Check sheet for the drawn part. Datum: minimum x, y, z corner. Units: mm. A direction names the side the tool comes from. Round coordinates to 2 decimals unless told otherwise and drop trailing zeros. Write each loop counter-clockwise with the first axis right and the second up, starting at its lowest first coordinate (ties: lowest second). Pieces come first, ordered by that corner, then holes. Notation, with made-up numbers: (3.5, 86.5) - (9.5, 86.5) arc R19 cw to (9.5, 117.5) - close; hole circle Ø5 at (15, 6.5). An arc over 180 degrees is marked (long way). Answer as a JSON object with one key per item and string values.
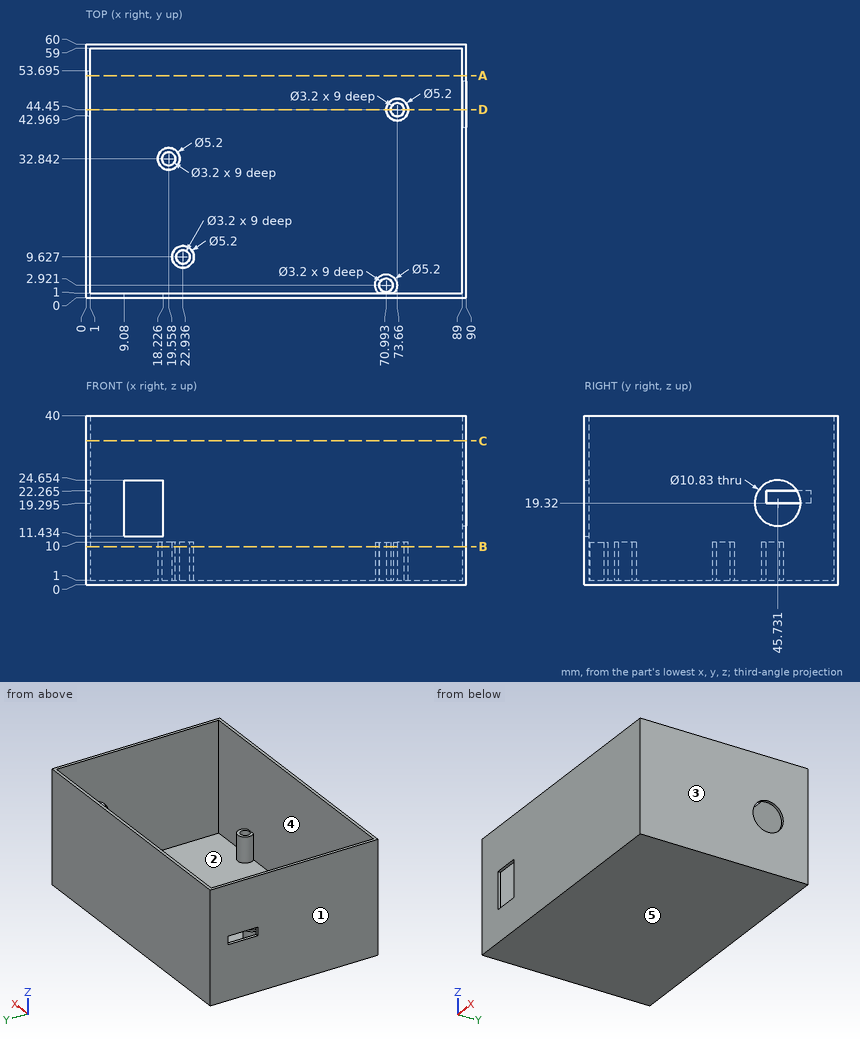
1. Mould release check, pull along X, two halves, no side actions. Record for the marked faces 1, 2 and 3: released by +X, released by -X, zero draft, split by the parting line, or undercut.
Completed:
{"face 1": "released by -X", "face 2": "undercut", "face 3": "released by +X"}
2. Cross-section at B-B (z = 9). Count the separate pieces of the cut face and the enclosed holes in it.
Completed:
{"separate pieces": "4", "enclosed holes": "5"}
3. Go/stop test with flat-tipped pins: pin 1 (1 mm diameter, centred on x = 71.5, y = 3.5, fed in from +Z); pin 2 (9.5 mm diameter, centred on y = 45.73, z = 19.32, fed in from +X). Record where each tip stops, or that it passes through.
Completed:
{"pin 1": "stops at z = 1", "pin 2": "stops at x = 1"}
4. Material ranges on probe 1 along Y at (x, z) = (73.66, 7); probe 2 along X at (y, z) = (51, 11.5); probe 3 along Y at (x, z) = (21, 13.5), recorded low to high. Write a range as from..to.
Completed:
{"probe 1": "y = 0..1, 41.85..42.85, 46.05..47.05, 59..60", "probe 2": "x = 0..1, 89..90", "probe 3": "y = 0..1, 59..60"}
5. Cross-section at D-D (y = 44.45). Record the boundary of the cut face in (x, z) (1 decimal).
Completed:
{"outline": "(0, 0) - (90, 0) - (90, 14.1) - (89, 14.1) - (89, 1) - (76.3, 1) - (76.3, 10) - (75.3, 10) - (75.3, 1) - (72.1, 1) - (72.1, 10) - (71.1, 10) - (71.1, 1) - (1, 1) - (1, 19.3) - (0, 19.3) - close; (0, 22.3) - (1, 22.3) - (1, 40) - (0, 40) - close; (89, 24.6) - (90, 24.6) - (90, 40) - (89, 40) - close"}
6. Access from +Z, -Z, +X, -X, +Y, -Y to the whole of each face (thin tool, end or side, straight path). Record for the marked faces 4 and 5.
Completed:
{"face 4": "+Z", "face 5": "-Z, +X, -X, +Y, -Y"}
7. Cross-section at A-A (y = 52.5). Record the boundary of the cut face in (x, z) (1 decimal), plus the area to 3 significant figures.
Completed:
{"outline": "(0, 0) - (90, 0) - (90, 40) - (89, 40) - (89, 1) - (1, 1) - (1, 19.3) - (0, 19.3) - close; (0, 22.3) - (1, 22.3) - (1, 40) - (0, 40) - close", "area": "165 mm^2"}
8. Cross-section at C-C (z = 34). Record the boundary of the cut face in (x, y).
Completed:
{"outline": "(0, 0) - (90, 0) - (90, 60) - (0, 60) - close; hole (1, 1) - (89, 1) - (89, 59) - (1, 59) - close"}
